```python
from build123d import *

# Parameters (mm, degrees)
CHAMFER1_SIZE = 0.1


with BuildPart() as part:
    # Sketch1 → Revolve1 (revolve)
    with BuildSketch(Plane(origin=(0, 0, 0), x_dir=(0, 0, -1), z_dir=(1, 0, 0))):
        Polygon((5, -1), (5, 2), (4.099649114, 2), (4.049649114, 1.9), (3.999649114, 2), (2.500350886, 2), (2.450350886, 1.9), (2.400350886, 2), (1.5, 2), (1.5, -2), (2.400350886, -2), (2.450350886, -1.9), (2.500350886, -2), (3.999649114, -2), (4.049649114, -1.9), (4.099649114, -2), (5.75, -2), (5.75, -1), align=None)
    revolve(axis=Axis((0, -2, 0), (0, 1, 0)))

    # Chamfer1
    chamfer1_edges = [part.edges().sort_by_distance(p)[0] for p in [
        (0, 2, 1.5),
        (0, 2, 5),
        (0, -2, 1.5),
    ]]
    chamfer(chamfer1_edges, length=CHAMFER1_SIZE)


solid = part.part
```
Model file for the job. Use its own axes, mm. A direction names the side the tool comes from. Coordinates: 2 decimals unless noted, no trailing zeros. Order: outer loops, then holes, each group sorted by start corner. A loop starts at its lowest first (then second) coordinate and runs counter-clockwise, first axis right, second up. Notation, with made-up numbers: (73.25, 37) - (94.25, 37) arc R29 cw to (94.25, 61) - close; hole circle Ø2 at (41.25, 59). An arc over 180 degrees is marked (long way). Return JSON: item names as keys, results as strings. Group by question number.
1) Mould opens along X. For faces 3 (the flat face through (4, -2, 2)), 4 (the cylindrical face through (4.88, 0.47, 1.08)), 5 (the cylindrical face through (-0.07, -0.03, 1.5)) say: released by +X, released by -X, zero draft, split by the parting line, or undercut.
2) Probe line 1 (Z direction, x = 0, y = -0.3); line 2 (X direction, y = -1.05, z = 0). List the from-to ranges inside material, lowest first. Write a range as from..to.
3) Saw through at A-A, the plane y = -0.65. Write the cut outline in (x, z).
4) Flat gauge pins, fed straight in: P1, Ø3, axis at x = 0.5, z = -0.5, coming from the -Y side; P2, Ø1.8, axis at x = 0, z = 0, coming from the -Y side. Where does each tip first touch, or does it go through?
5) Tool access for faces 1 (the flat face through (2, -2, -2)), 2 (the flat face through (-5, -1, 2)): list every direction of +Z, -Z, +X, -X, +Y, -Y with a clear straight run to the whole face (end or side of a thin tool).
Values found:
{
 "1": {"face 3": "zero draft", "face 4": "split by the parting line", "face 5": "undercut"},
 "2": {"line 1": "z = -5..-1.5, 1.5..5", "line 2": "x = -5.75..-1.5, 1.5..5.75"},
 "3": {"outline": "circle Ø10 at (0, 0); hole circle Ø3 at (0, 0)"},
 "4": {"P1": "stops at y = -2", "P2": "passes through"},
 "5": {"face 1": "+Z, -Z, +X, -X, -Y", "face 2": "+Y"}
}
